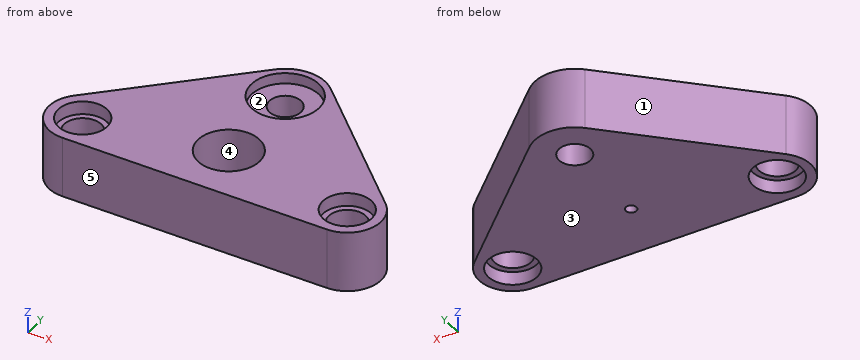
from build123d import *

# Parameters (mm, degrees)
SKETCH1_R           = 5.175
SKETCH1_R_2         = 6.075
BOSS_EXTRUDE1_DEPTH = 20
SKETCH2_R           = 11.075
CUT_EXTRUDE1_DEPTH  = 3.55
SKETCH3_R           = 8
CUT_EXTRUDE2_DEPTH  = 4.35
CUT_EXTRUDE3_START  = -4.35
SKETCH4_R           = 8
CUT_EXTRUDE3_DEPTH  = 4.35
SKETCH5_R           = 10.075
CUT_EXTRUDE4_DEPTH  = 15
SKETCH6_R           = 1.75
CUT_EXTRUDE5_DEPTH  = 5


with BuildPart() as part:
    # Sketch1 → Boss-Extrude1 (new body)
    with BuildSketch(Plane.XY):
        with BuildLine():
            Line((9.091765785, 9.535219972), (50.642603876, -30.08321455))
            ThreePointArc((50.642603876, -30.08321455), (53.281680295, -42.214737327), (43, -49.173589213))
            Line((43, -49.173589213), (-43, -49.173589213))
            ThreePointArc((-43, -49.173589213), (-53.281680295, -42.214737327), (-50.642603876, -30.08321455))
            Line((-50.642603876, -30.08321455), (-9.091765785, 9.535219972))
            ThreePointArc((-9.091765785, 9.535219972), (0, 13.175), (9.091765785, 9.535219972))
        make_face()
        Circle(SKETCH1_R, mode=Mode.SUBTRACT)
        with Locations((43, -38.098589213)):
            Circle(SKETCH1_R_2, mode=Mode.SUBTRACT)
        with Locations((-43, -38.098589213)):
            Circle(SKETCH1_R_2, mode=Mode.SUBTRACT)
    extrude(amount=BOSS_EXTRUDE1_DEPTH)

    # Sketch2 → Cut-Extrude1 (cut)
    with BuildSketch(Plane.XY.offset(20)):
        Circle(SKETCH2_R)
    extrude(amount=-CUT_EXTRUDE1_DEPTH, mode=Mode.SUBTRACT)

    # Sketch3 → Cut-Extrude2 (cut)
    with BuildSketch(Plane(origin=(0, 0, 0), x_dir=(-1, 0, 0), z_dir=(0, 0, -1))):
        with Locations((43, -38.098589213)):
            Circle(SKETCH3_R)
        with Locations((-43, -38.098589213)):
            Circle(SKETCH3_R)
    extrude(amount=-CUT_EXTRUDE2_DEPTH, mode=Mode.SUBTRACT)

    # Sketch4 → Cut-Extrude3 (cut)
    with BuildSketch(Plane.XY.offset(20).offset(CUT_EXTRUDE3_START)):
        with Locations(Location((-43, -38.098589213, 0), (0, 0, 180))):
            Circle(SKETCH4_R)
        with Locations(Location((43, -38.098589213, 0), (0, 0, 180))):
            Circle(SKETCH4_R)
    extrude(amount=CUT_EXTRUDE3_DEPTH, mode=Mode.SUBTRACT)

    # Sketch5 → Cut-Extrude4 (cut)
    with BuildSketch(Plane.XY.offset(20)):
        with Locations((0, -30.593589213)):
            Circle(SKETCH5_R)
    extrude(amount=-CUT_EXTRUDE4_DEPTH, mode=Mode.SUBTRACT)

    # Sketch6 → Cut-Extrude5 (cut)
    with BuildSketch(Plane.XY.offset(5)):
        with Locations((0, -30.593589213)):
            Circle(SKETCH6_R)
    extrude(amount=-CUT_EXTRUDE5_DEPTH, mode=Mode.SUBTRACT)


solid = part.part
Input: part model. Units: mm. Frame: model coordinates. Face numbers are marked on the shaded views. A direction names the side the tool comes from. Coordinates: 2 decimals unless noted, no trailing zeros. Loops run counter-clockwise (first coordinate to the right, second up) from the corner with the lowest first, then second, coordinate; pieces in that order, holes last.
Q1. Cut plane B-B (y = 0). Output: boundary loops of the cut face in (x, z) (3 decimals).
Q2. Draft query along Z for the marked faces 1, 2 and 3. Return one class per face: +Z half, -Z half, draft (parallel to the pull), parting line (faces both ways), or undercut.
Q3. Cut plane C-C (x = -38.5). Output: boundary loops of the cut face in (y, z).
Q4. Contact query for flat-ended pins moving along their axis: pin 1 (1.5 mm diameter, centred on x = -15, z = 12.5, fed in from +Y); pin 2 (13 mm diameter, centred on x = -43, y = -38.1, fed in from +Z); pin 3 (10 mm diameter, centred on x = -19.5, z = 5, fed in from +Y). Output: stop coordinate, or through.
Q5. Cut plane D-D (z = 9.25). Output: boundary loops of the cut face in (x, y) (3 decimals).
Q6. Material intervals for line 1 (Y direction, x = 0, z = 11.5) (3 decimals); line 2 (Y direction, x = 0, z = 18.6) (3 decimals); line 3 (X direction, y = -41, z = 11.5), sorted ascending.
Q7. Set-up query: the marked faces 4 and 5. Return all of +Z, -Z, +X, -X, +Y, -Y with unobstructed straight access to the full face (end or side cutting, diameter ignored); none if empty.
Q8. Cut plane A-A (x = 0). Output: boundary loops of the cut face in (y, z) (3 decimals), then the cut area to 3 significant figures.
Working result:
1. outline: (-19.092, 0) - (-5.175, 0) - (-5.175, 16.45) - (-11.075, 16.45) - (-11.075, 20) - (-19.092, 20) - close; (5.175, 0) - (19.092, 0) - (19.092, 20) - (11.075, 20) - (11.075, 16.45) - (5.175, 16.45) - close
2. face 1: draft
2. face 2: +Z half
2. face 3: -Z half
3. outline: (-49.17, 0) - (-44.71, 0) - (-44.71, 4.35) - (-42.18, 4.35) - (-42.18, 15.65) - (-44.71, 15.65) - (-44.71, 20) - (-49.17, 20) - close; (-34.02, 4.35) - (-31.48, 4.35) - (-31.48, 0) - (-18.51, 0) - (-18.51, 20) - (-31.48, 20) - (-31.48, 15.65) - (-34.02, 15.65) - close
4. pin 1: stops at y = 4.62
4. pin 2: stops at z = 15.65
4. pin 3: stops at y = 4.38
5. outline: (-50.643, -30.083) arc R11.075 ccw to (-43, -49.174) - (43, -49.174) arc R11.075 ccw to (50.643, -30.083) - (9.092, 9.535) arc R13.175 ccw to (-9.092, 9.535) - close; hole circle Ø12.15 at (-43, -38.099); hole circle Ø20.15 at (0, -30.594); hole circle Ø10.35 at (0, 0); hole circle Ø12.15 at (43, -38.099)
6. line 1: y = -49.174 to -40.669, -20.519 to -5.175, 5.175 to 13.175
6. line 2: y = -49.174 to -40.669, -20.519 to -11.075, 11.075 to 13.175
6. line 3: x = -53.69 to -48.34, -37.66 to 37.66, 48.34 to 53.69
7. face 4: +Z
7. face 5: +Z, -Z, +X, -X, -Y
8. outline: (-49.174, 0) - (-32.344, 0) - (-32.344, 5) - (-40.669, 5) - (-40.669, 20) - (-49.174, 20) - close; (-28.844, 0) - (-5.175, 0) - (-5.175, 16.45) - (-11.075, 16.45) - (-11.075, 20) - (-20.519, 20) - (-20.519, 5) - (-28.844, 5) - close; (5.175, 0) - (13.175, 0) - (13.175, 20) - (11.075, 20) - (11.075, 16.45) - (5.175, 16.45) - close
8. area: 678 mm2
